The listing builds one solid part. Answer for the finished solid, in the listing's coordinates (mm). Round coordinates to 2 decimals unless told otherwise and drop trailing zeros. Order: outer loops, then holes, each group sorted by start corner. A loop starts at its lowest first (then second) coordinate and runs counter-clockwise, first axis right, second up. Notation, with made-up numbers: (54.25, -3.5) -> (99.25, -3.5) arc R14 ccw to (99.25, 3.5) -> close; hole circle Ø2 at (33.25, 79.25). An arc over 180 degrees is marked (long way). Return JSON: item names as keys, results as strings. Group by question number.
(1) Each of these flat-tipped pins is pushed along its axis until it touches: pin 1 (9 mm diameter, centred on x = 148.49, y = -148.49, fed in from -Z); pin 2 (5 mm diameter, centred on y = -152, z = 3, fed in from +X); pin 3 (5 mm diameter, centred on x = 100, z = 8, fed in from -Y); pin 4 (1.5 mm diameter, centred on x = -128, z = 7.5, fed in from +Y). Where does it stop, or does it pass through?
(2) The part is cut by section A-A (z = 5). Count the separate pieces of the cut face and the enclosed holes in it, plus the area to 3 significant figures.
(3) The part is cut by section B-B (y = 96). Determine the outline of the cut face in (x, z).
(4) Consider line 1 (Y direction, x = 0, z = 3); line 2 (Y direction, x = 52.5, z = 7.25); line 3 (Y direction, x = 12.5, z = 0.75). Determine where each line is inside the solid, lowest interval first. Write a range as [from, to].
(5) Determine the mould class of faces 1 (the face through (-59, -52, 0)), 2 (the face through (-249.76, 10.99, 5.42)), 3 (the face through (-9.764, 74.362, 5.423)) for opening direction Y: +Y half, -Y half, draft (parallel to the pull), parting line (faces both ways), or undercut.
from build123d import *

# Parameters (mm, degrees)
SKETCH2_R           = 250
SKETCH2_R_2         = 75
BOSS_EXTRUDE1_DEPTH = 11
SKETCH3_R           = 5
CUT_EXTRUDE1_DEPTH  = 354.724469043


with BuildPart() as part:
    # Sketch2 → Boss-Extrude1 (new body)
    with BuildSketch(Plane.XY):
        Circle(SKETCH2_R)
        Circle(SKETCH2_R_2, mode=Mode.SUBTRACT)
    extrude(amount=BOSS_EXTRUDE1_DEPTH)

    # Sketch3 → Cut-Extrude1 (cut, through all)
    with BuildSketch(Plane.XY.offset(11)):
        with Locations((0, 210)):
            Circle(SKETCH3_R)
        with Locations((148.492424049, 148.492424049)):
            Circle(SKETCH3_R)
        with Locations((210, 0)):
            Circle(SKETCH3_R)
        with Locations((148.492424049, -148.492424049)):
            Circle(SKETCH3_R)
        with Locations((0, -210)):
            Circle(SKETCH3_R)
        with Locations((-148.492424049, -148.492424049)):
            Circle(SKETCH3_R)
        with Locations((-210, 0)):
            Circle(SKETCH3_R)
        with Locations((-148.492424049, 148.492424049)):
            Circle(SKETCH3_R)
    extrude(amount=-CUT_EXTRUDE1_DEPTH, mode=Mode.SUBTRACT)


solid = part.part
Answer below:
{
 "1": {"pin 1": "passes through", "pin 2": "stops at x = 200.37", "pin 3": "stops at y = -230.2", "pin 4": "stops at y = 215.19"},
 "2": {"separate pieces": "1", "enclosed holes": "9", "area": "178,000 mm²"},
 "3": {"outline": "(-230.83, 0) -> (230.83, 0) -> (230.83, 11) -> (-230.83, 11) -> close"},
 "4": {"line 1": "y = [-250, -215], [-205, -75], [75, 205], [215, 250]", "line 2": "y = [-244.43, -53.56], [53.56, 244.43]", "line 3": "y = [-249.69, -73.95], [73.95, 249.69]"},
 "5": {"face 1": "draft", "face 2": "parting line", "face 3": "undercut"}
}
